```python
from build123d import *

# Parameters (mm, degrees)
SKETCH_1_W                 = 300
SKETCH_1_H                 = 12
EXTRUDE_268_DEPTH          = 18.35
HOLE_WIZARD_M4_D           = 5.5
HOLE_WIZARD_M4_CSINK_D     = 10.4
HOLE_WIZARD_M4_CSINK_ANGLE = 90
PATTERN_LINEAR_1_COUNT     = 3
PATTERN_LINEAR_1_PITCH     = 60
PATTERN_LINEAR_1_COL_COUNT = 3
PATTERN_LINEAR_1_COL_PITCH = 60
SKETCH_5_R                 = 3
CUT_EXTRUDE_6_DEPTH        = 11


with BuildPart() as part:
    # Эскиз1 → Extrude 268 (new body)
    with BuildSketch(Plane(origin=(0, 0, 0), x_dir=(1, 0, 0), z_dir=(0, 1, 0))):
        with Locations((0, 6)):
            Rectangle(SKETCH_1_W, SKETCH_1_H)
    extrude(amount=EXTRUDE_268_DEPTH)

    # Крепление-M4 (through all)
    with Locations(Plane(origin=(0, 18.35, 0), x_dir=(-1, 0, 0), z_dir=(0, 1, 0))):
        with Locations((0, -6)):
            hole_wizard_m4 = CounterSinkHole(HOLE_WIZARD_M4_D / 2, HOLE_WIZARD_M4_CSINK_D / 2, counter_sink_angle=HOLE_WIZARD_M4_CSINK_ANGLE)

    # Линейный массив1: Крепление-M4 ×3
    with Locations(*[(-i * PATTERN_LINEAR_1_PITCH, 0, 0) for i in range(1, PATTERN_LINEAR_1_COUNT)]):
        add(hole_wizard_m4, mode=Mode.SUBTRACT)

    # Линейный массив1 col: Крепление-M4 ×3
    with Locations(*[(i * PATTERN_LINEAR_1_COL_PITCH, 0, 0) for i in range(1, PATTERN_LINEAR_1_COL_COUNT)]):
        add(hole_wizard_m4, mode=Mode.SUBTRACT)

    # Эскиз5 → Валы-6мм (cut)
    with BuildSketch(Plane.XY.offset(-12)):
        with Locations((-144, 9.175)):
            Circle(SKETCH_5_R)
        with Locations((144, 9.175)):
            Circle(SKETCH_5_R)
    extrude(amount=CUT_EXTRUDE_6_DEPTH, mode=Mode.SUBTRACT)


solid = part.part
```
CAD build for the part. Positions are in the model's coordinates, mm. A direction names the side the tool comes from. Round coordinates to 2 decimals unless told otherwise and drop trailing zeros. Write each loop counter-clockwise with the first axis right and the second up, starting at its lowest first coordinate (ties: lowest second). Pieces come first, ordered by that corner, then holes. Notation, with made-up numbers: (85.25, -27) - (132.25, -27) arc R27 cw to (132.25, 0) - close; hole circle Ø10 at (-11.75, 82.25). An arc over 180 degrees is marked (long way). Return JSON: item names as keys, results as strings. Group by question number.
Item 1: Band-saw the part on B-B on x = -144. List the corners of the cut face in (y, z) (3 decimals), plus the area to 3 significant figures.
Item 2: Probe probe 1 along X at (y, z) = (5.5, -6); probe 2 along Y at (x, z) = (-144, -8.5) (3 decimals); probe 3 along Z at (x, y) = (0, 9). List the from-to ranges inside material, lowest first.
Item 3: Band-saw the part on C-C on z = -6. State how many separate pieces and enclosed holes the cut face has, plus the area to 3 significant figures.
Item 4: Band-saw the part on A-A on x = 0. List the corners of the cut face in (y, z).
Item 5: 3-axis set-ups, long thin cutter, end or side, ignore diameter. For faces 1 (the face through (-62.866, 16.019, -5.874)), 2 (the face through (146.86, 10.08, -6.58)): which of +Z, -Z, +X, -X, +Y, -Y reach the whole face in a straight line?
Item 6: Mould opens along Y. For faces 3 (the face through (-144, 9, -1)), 4 (the face through (117.134, 16.019, -5.874)), 5 (the face through (119.404, 7.839, -8.685)), 6 (the face through (144, 9, -1)) say: +Y half, -Y half, draft (parallel to the pull), parting line (faces both ways), or undercut.
Item 7: Flat gauge pins, fed straight in: pin 1 Ø6.5 at (x, z) = (120, -6) entering from +Y; pin 2 Ø3.5 at (x, z) = (60, -6) entering from -Y; pin 3 Ø1.8 at (x, y) = (-144, 10.5) entering from -Z. Where does each tip first touch, or does it go through?
Resolved:
{
 "1": {"outline": "(0, -12) - (6.175, -12) - (6.175, -1) - (12.175, -1) - (12.175, -12) - (18.35, -12) - (18.35, 0) - (0, 0) - close", "area": "154 mm²"},
 "2": {"probe 1": "x = -150 to -122.75, -117.25 to -62.75, -57.25 to -2.75, 2.75 to 57.25, 62.75 to 117.25, 122.75 to 150", "probe 2": "y = 0 to 6.175, 12.175 to 18.35", "probe 3": "z = -12 to -8.75, -3.25 to 0"},
 "3": {"separate pieces": "6", "enclosed holes": "2", "area": "4,910 mm²"},
 "4": {"outline": "(0, -12) - (18.35, -12) - (18.35, -11.2) - (15.9, -8.75) - (0, -8.75) - close; (0, -3.25) - (15.9, -3.25) - (18.35, -0.8) - (18.35, 0) - (0, 0) - close"},
 "5": {"face 1": "+Y", "face 2": "-Z"},
 "6": {"face 3": "undercut", "face 4": "+Y half", "face 5": "draft", "face 6": "undercut"},
 "7": {"pin 1": "stops at y = 16.4", "pin 2": "passes through", "pin 3": "stops at z = -1"}
}
